Geometry check sheet. Reference: the model listing, model coordinates, mm. Face numbers are marked on the shaded views. A direction names the side the tool comes from. Give positions to 0.01 mm unless a question says otherwise; leave off trailing zeros. Loops run counter-clockwise (first coordinate to the right, second up) from the corner with the lowest first, then second, coordinate; pieces in that order, holes last.
1. Cross-section at B-B, the plane x = -24. Record the cut outline in (y, z).
2. Go/stop test with flat-tipped pins: pin 1 Ø1 at (x, z) = (-52, -0.5) entering from +Y; pin 2 Ø1.9 at (x, z) = (18.5, -3.5) entering from -Y; pin 3 Ø1.5 at (x, z) = (3.5, -14.5) entering from -Y; pin 4 Ø4 at (x, y) = (52.39, 0) entering from +Z. Record where each tip stops, or that it passes through.
3. Tool access check on the marked faces 3 and 4. Record the directions out of +Z, -Z, +X, -X, +Y, -Y that give a thin tool (end or side, any length) a straight path to the whole face; none if there is none.
4. Release check for a two-part mould opening along Z. For the marked faces 1 and 2 record: +Z half, -Z half, draft (parallel to the pull), parting line (faces both ways), or undercut.
5. Cross-section at A-A, the plane y = 0. Record the cut outline in (x, z), plus the area to 3 significant figures.
6. Material ranges on L1, parallel to Y at x = 3, z = -4; L2, parallel to Z at x = 40, y = 0; L3, parallel to Y at x = 33.5, z = -5.75, recorded low to high.
from build123d import *

# Parameters (mm, degrees)
SKETCH1_W                                 = 0.91186
SKETCH1_H                                 = 6.731
BASE_FLANGE1_DEPTH                        = 57.15
EDGE_FLANGE1_DEPTH                        = 101.6
EDGE_FLANGE2_DEPTH                        = 101.6
EDGE_FLANGE3_DEPTH                        = 101.6
CUT_EXTRUDE1_START                        = -2.539504
SKETCH21_W                                = 63.5
SKETCH21_H                                = 12.718519465
CUT_EXTRUDE1_DEPTH                        = 2.836243
EDGE_FLANGE4_DEPTH                        = 60.325
EDGE_FLANGE5_DEPTH                        = 25.4
EDGE_FLANGE6_DEPTH                        = 25.4
BREAK_CORNER3_START                       = 0.436452344
BREAK_CORNER3_DEPTH                       = 0.91186
BREAK_CORNER3_START_2                     = -1.348312344
BREAK_CORNER3_2_DEPTH                     = 0.91186
BREAK_CORNER4_START                       = -5.26796
BREAK_CORNER4_DEPTH                       = 0.91186
BREAK_CORNER4_START_2                     = -0.91186
BREAK_CORNER4_2_DEPTH                     = 0.91186
HOLE_FOR_M3_FLUSH_HEAD_STUDS_FH_FHS_FHA_D = 3


# Read off the part's stored shape, not the designer's step: Break-Corner3, Break-Corner4
# Sheet-metal steps are written as plain solids
with BuildPart() as part:
    # Sketch1 → Base-Flange1 (new, symmetric)
    with BuildSketch(Plane(origin=(0, 0, 0), x_dir=(0, 0, -1), z_dir=(1, 0, 0))):
        with Locations((0.45593, 0)):
            Rectangle(SKETCH1_W, SKETCH1_H)
    extrude(amount=BASE_FLANGE1_DEPTH, both=True)

    # Edge-Flange1 section (across the edge) → Edge-Flange1 (add)
    with BuildSketch(Plane(origin=(-50.8, 4.3561, -0.91186), x_dir=(0, -1, 0), z_dir=(1, 0, 0))):
        with BuildLine():
            Line((-0.91186, 0.9906), (-0.91186, 4.75234))
            Line((-0.91186, 4.75234), (0, 4.75234))
            Line((0, 4.75234), (0, 0.9906))
            ThreePointArc((0, 0.9906), (0.290140023, 0.290140023), (0.9906, 0))
            Line((0.9906, 0), (0.9906, -0.91186))
            ThreePointArc((0.9906, -0.91186), (-0.354642367, -0.354642367), (-0.91186, 0.9906))
        make_face()
    extrude(amount=EDGE_FLANGE1_DEPTH)

    # Edge-Flange2 section (across the edge) → Edge-Flange2 (add)
    with BuildSketch(Plane(origin=(-50.8, 4.3561, -5.803419751), x_dir=(0, -0.9612616959383217, 0.27563735581698934), z_dir=(1, 0, 0))):
        with BuildLine():
            Line((-0.91186, 0.139219751), (-0.91186, 5.637646434))
            Line((-0.91186, 5.637646434), (0, 5.637646434))
            Line((0, 5.637646434), (0, 0.139219751))
            ThreePointArc((0, 0.139219751), (0.009640451, 0.001354877), (0.038374164, -0.133826614))
            Line((0.038374164, -0.133826614), (-0.838161926, -0.385169293))
            ThreePointArc((-0.838161926, -0.385169293), (-0.89334539, -0.125551507), (-0.91186, 0.139219751))
        make_face()
    extrude(amount=EDGE_FLANGE2_DEPTH)

    # Edge-Flange3 section (across the edge) → Edge-Flange3 (add)
    with BuildSketch(Plane(origin=(50.8, 3.592598946, -11.774251656), x_dir=(0, 0.9455185755993153, 0.32556815445716125), z_dir=(-1, 0, 0))):
        with BuildLine():
            Line((-0.91186, 0.31233498), (-0.91186, 6.057411646))
            Line((-0.91186, 6.057411646), (0, 6.057411646))
            Line((0, 6.057411646), (0, 0.31233498))
            ThreePointArc((0, 0.31233498), (0.045847989, 0.014455815), (0.179147985, -0.255849838))
            Line((0.179147985, -0.255849838), (-0.567803998, -0.778871247))
            ThreePointArc((-0.567803998, -0.778871247), (-0.82380835, -0.259745775), (-0.91186, 0.31233498))
        make_face()
    extrude(amount=EDGE_FLANGE3_DEPTH)

    # Sketch21 → Cut-Extrude1 (cut)
    with BuildSketch(Plane(origin=(0, 5.26796, 0), x_dir=(1, 0, 0), z_dir=(0, 1, 0)).offset(CUT_EXTRUDE1_START)):
        with Locations((0, 11.439259733)):
            Rectangle(SKETCH21_W, SKETCH21_H)
    extrude(amount=CUT_EXTRUDE1_DEPTH, mode=Mode.SUBTRACT)

    # Edge-Flange4 section (across the edge) → Edge-Flange4 (add)
    with BuildSketch(Plane(origin=(30.1625, -4.3561, -0.91186), x_dir=(0, 1, 0), z_dir=(-1, 0, 0))):
        with BuildLine():
            Line((-0.91186, 0.9906), (-0.91186, 4.16814))
            Line((-0.91186, 4.16814), (0, 4.16814))
            Line((0, 4.16814), (0, 0.9906))
            ThreePointArc((0, 0.9906), (0.290140023, 0.290140023), (0.9906, 0))
            Line((0.9906, 0), (0.9906, -0.91186))
            ThreePointArc((0.9906, -0.91186), (-0.354642367, -0.354642367), (-0.91186, 0.9906))
        make_face()
    extrude(amount=EDGE_FLANGE4_DEPTH)

    # Edge-Flange5 section (across the edge) → Edge-Flange5 (add)
    with BuildSketch(Plane(origin=(12.7, -4.3561, -5.803419751), x_dir=(0, 0.9612616959383217, 0.27563735581698967), z_dir=(-1, 0, 0))):
        with BuildLine():
            Line((-0.91186, 0.139219751), (-0.91186, 5.637646434))
            Line((-0.91186, 5.637646434), (0, 5.637646434))
            Line((0, 5.637646434), (0, 0.139219751))
            ThreePointArc((0, 0.139219751), (0.009640451, 0.001354877), (0.038374164, -0.133826614))
            Line((0.038374164, -0.133826614), (0.199401507, -0.695395697))
            Line((0.199401507, -0.695395697), (-0.677134583, -0.946738376))
            Line((-0.677134583, -0.946738376), (-0.838161926, -0.385169293))
            ThreePointArc((-0.838161926, -0.385169293), (-0.89334539, -0.125551507), (-0.91186, 0.139219751))
        make_face()
    extrude(amount=EDGE_FLANGE5_DEPTH)

    # Edge-Flange6 section (across the edge) → Edge-Flange6 (add)
    with BuildSketch(Plane(origin=(-12.7, -3.592598946, -11.774251656), x_dir=(0, -0.9455185755993154, 0.325568154457161), z_dir=(1, 0, 0))):
        with BuildLine():
            Line((-0.91186, 0.31233498), (-0.91186, 6.062491646))
            Line((-0.91186, 6.062491646), (0, 6.062491646))
            Line((0, 6.062491646), (0, 0.31233498))
            ThreePointArc((0, 0.31233498), (0.045847989, 0.014455815), (0.179147985, -0.255849838))
            Line((0.179147985, -0.255849838), (-0.567803998, -0.778871247))
            ThreePointArc((-0.567803998, -0.778871247), (-0.82380835, -0.259745775), (-0.91186, 0.31233498))
        make_face()
    extrude(amount=EDGE_FLANGE6_DEPTH)

    # Break-Corner3 outline → Break-Corner3 (cut)
    with BuildSketch(Plane(origin=(0, 0, 0), x_dir=(1, 0, 0), z_dir=(0, 0.9455185755993153, -0.3255681544571611)).offset(BREAK_CORNER3_START)):
        with BuildLine():
            Line((12.7, 18.364901109), (9.525, 18.364901109))
            ThreePointArc((9.525, 18.364901109), (11.77006403, 17.434965139), (12.7, 15.189901109))
            Line((12.7, 15.189901109), (12.7, 18.364901109))
        make_face()
        with BuildLine():
            ThreePointArc((-12.7, 15.189901109), (-11.77006403, 17.434965139), (-9.525, 18.364901109))
            Line((-9.525, 18.364901109), (-12.7, 18.364901109))
            Line((-12.7, 18.364901109), (-12.7, 15.189901109))
        make_face()
    extrude(amount=BREAK_CORNER3_DEPTH, mode=Mode.SUBTRACT)

    # Break-Corner3 2 outline → Break-Corner3 2 (cut)
    with BuildSketch(Plane(origin=(0, 0, 0), x_dir=(1, 0, 0), z_dir=(0, 0.9455185755993153, 0.3255681544571611)).offset(BREAK_CORNER3_START_2)):
        with BuildLine():
            ThreePointArc((-50.8, 15.184821109), (-49.87006403, 17.429885139), (-47.625, 18.359821109))
            Line((-47.625, 18.359821109), (-50.8, 18.359821109))
            Line((-50.8, 18.359821109), (-50.8, 15.184821109))
        make_face()
        with BuildLine():
            Line((-31.75, 18.359821109), (-34.925, 18.359821109))
            ThreePointArc((-34.925, 18.359821109), (-32.67993597, 17.429885139), (-31.75, 15.184821109))
            Line((-31.75, 15.184821109), (-31.75, 18.359821109))
        make_face()
        with BuildLine():
            Line((31.75, 18.359821109), (31.75, 15.184821109))
            ThreePointArc((31.75, 15.184821109), (32.67993597, 17.429885139), (34.925, 18.359821109))
            Line((34.925, 18.359821109), (31.75, 18.359821109))
        make_face()
        with BuildLine():
            Line((50.8, 18.359821109), (47.625, 18.359821109))
            ThreePointArc((47.625, 18.359821109), (49.87006403, 17.429885139), (50.8, 15.184821109))
            Line((50.8, 15.184821109), (50.8, 18.359821109))
        make_face()
    extrude(amount=BREAK_CORNER3_2_DEPTH, mode=Mode.SUBTRACT)

    # Break-Corner4 outline → Break-Corner4 (cut)
    with BuildSketch(Plane(origin=(0, 0, 0), x_dir=(1, 0, 0), z_dir=(0, 1, 0)).offset(BREAK_CORNER4_START)):
        with BuildLine():
            ThreePointArc((28.575, 5.08), (29.697532015, 4.615032015), (30.1625, 3.4925))
            Line((30.1625, 3.4925), (30.1625, 5.08))
            Line((30.1625, 5.08), (28.575, 5.08))
        make_face()
        with BuildLine():
            ThreePointArc((-30.1625, 3.4925), (-29.697532015, 4.615032015), (-28.575, 5.08))
            Line((-28.575, 5.08), (-30.1625, 5.08))
            Line((-30.1625, 5.08), (-30.1625, 3.4925))
        make_face()
    extrude(amount=BREAK_CORNER4_DEPTH, mode=Mode.SUBTRACT)

    # Break-Corner4 2 outline → Break-Corner4 2 (cut)
    with BuildSketch(Plane.XY.offset(BREAK_CORNER4_START_2)):
        with BuildLine():
            Line((-57.15, 3.3655), (-57.15, 1.778))
            ThreePointArc((-57.15, 1.778), (-56.685032015, 2.900532015), (-55.5625, 3.3655))
            Line((-55.5625, 3.3655), (-57.15, 3.3655))
        make_face()
        with BuildLine():
            ThreePointArc((-55.5625, -3.3655), (-56.685032015, -2.900532015), (-57.15, -1.778))
            Line((-57.15, -1.778), (-57.15, -3.3655))
            Line((-57.15, -3.3655), (-55.5625, -3.3655))
        make_face()
        with BuildLine():
            Line((57.15, -3.3655), (57.15, -1.778))
            ThreePointArc((57.15, -1.778), (56.685032015, -2.900532015), (55.5625, -3.3655))
            Line((55.5625, -3.3655), (57.15, -3.3655))
        make_face()
        with BuildLine():
            ThreePointArc((55.5625, 3.3655), (56.685032015, 2.900532015), (57.15, 1.778))
            Line((57.15, 1.778), (57.15, 3.3655))
            Line((57.15, 3.3655), (55.5625, 3.3655))
        make_face()
    extrude(amount=BREAK_CORNER4_2_DEPTH, mode=Mode.SUBTRACT)

    # Hole for M3 Flush head Studs (FH,FHS,FHA,FH4)1 (through all)
    with Locations(Plane.XY):
        with Locations((52.3875, 0), (-52.3875, 0)):
            Hole(HOLE_FOR_M3_FLUSH_HEAD_STUDS_FH_FHS_FHA_D / 2)


solid = part.part
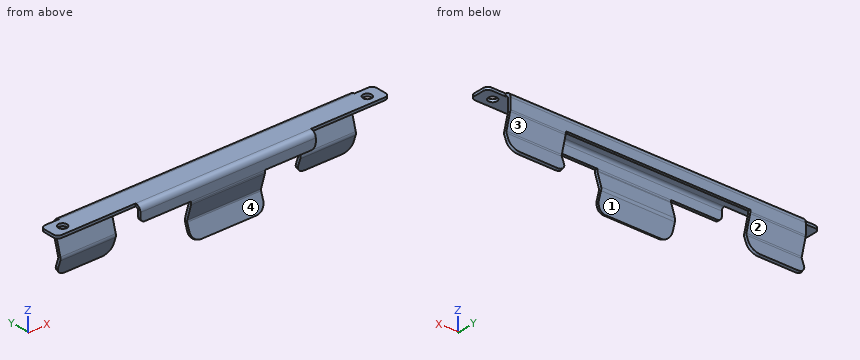
Result:
1. outline: (-5.27, -5.08) - (-4.36, -5.08) - (-4.36, -1.9) arc R0.99 cw to (-3.37, -0.91) - (3.37, -0.91) arc R0.99 cw to (4.36, -1.9) - (4.36, -5.08) - (5.27, -5.08) - (5.27, -1.9) arc R1.9 ccw to (3.37, 0) - (-3.37, 0) arc R1.9 ccw to (-5.27, -1.9) - close
2. pin 1: stops at y = 3.37
2. pin 2: stops at y = -5.27
2. pin 3: stops at y = -4.79
2. pin 4: stops at z = 0
3. face 3: +X, -X, +Y
3. face 4: +X, -X, -Y
4. face 1: -Z half
4. face 2: undercut
5. outline: (-57.15, -0.91) - (-53.89, -0.91) - (-53.89, 0) - (-57.15, 0) - close; (-50.89, -0.91) - (50.89, -0.91) - (50.89, 0) - (-50.89, 0) - close; (53.89, -0.91) - (57.15, -0.91) - (57.15, 0) - (53.89, 0) - close
5. area: 98.8 mm2
6. L1: y = -5.27 to -4.36, 4.36 to 5.27
6. L2: z = -0.91 to 0
6. L3: y = 4.35 to 5.27
